The model under review builds one solid part; all positions refer to its coordinate system, in mm. A direction names the side the tool comes from. Give positions to 0.01 mm unless a question says otherwise; leave off trailing zeros. Loops run counter-clockwise (first coordinate to the right, second up) from the corner with the lowest first, then second, coordinate; pieces in that order, holes last. Notation, with made-up numbers: (72.5, 37) - (108.5, 37) arc R28 ccw to (108.5, 68) - close; hole circle Ø2 at (40.25, 51). An arc over 180 degrees is marked (long way). Answer as a JSON object with one key per item and string values.
from build123d import *

# Parameters (mm, degrees)
SKETCH4_W            = 31.4
SKETCH4_H            = 31.4
SKETCH4_W_2          = 25.4
SKETCH4_H_2          = 25.4
BOSS_EXTRUDE3_DEPTH  = 30
SKETCH5_W            = 31.4
SKETCH5_H            = 31.4
BOSS_EXTRUDE4_DEPTH  = 5
SKETCH6_W            = 31.4
SKETCH6_H            = 8
BOSS_EXTRUDE5_DEPTH  = 5
BOSS_EXTRUDE6_DEPTH  = 8
SKETCH8_R            = 9.5
BOSS_EXTRUDE7_DEPTH  = 8
SKETCH9_W            = 31.4
SKETCH9_H            = 10
BOSS_EXTRUDE8_DEPTH  = 5
SKETCH10_W           = 31.4
SKETCH10_H           = 10
BOSS_EXTRUDE9_DEPTH  = 11
SKETCH11_W           = 5.2
SKETCH11_H           = 10
BOSS_EXTRUDE10_DEPTH = 40
BOSS_EXTRUDE11_DEPTH = 3
CUT_EXTRUDE1_START   = 8
SKETCH8_2_R          = 9.5
CUT_EXTRUDE1_DEPTH   = 24
SKETCH14_W           = 21
SKETCH14_H           = 13
CUT_EXTRUDE2_DEPTH   = 2


with BuildPart() as part:
    # Sketch4 → Boss-Extrude3 (new body)
    with BuildSketch(Plane.XY):
        Rectangle(SKETCH4_W, SKETCH4_H)
        Rectangle(SKETCH4_W_2, SKETCH4_H_2, mode=Mode.SUBTRACT)
    extrude(amount=BOSS_EXTRUDE3_DEPTH)

    # Sketch5 → Boss-Extrude4 (add)
    with BuildSketch(Plane.XY.offset(30)):
        Rectangle(SKETCH5_W, SKETCH5_H)
    extrude(amount=BOSS_EXTRUDE4_DEPTH)

    # Sketch6 → Boss-Extrude5 (add)
    with BuildSketch(Plane.XY.offset(35)):
        Rectangle(SKETCH6_W, SKETCH6_H)
    extrude(amount=BOSS_EXTRUDE5_DEPTH)

    # Sketch7 → Boss-Extrude6 (add)
    with BuildSketch(Plane.XZ.offset(4)):
        with BuildLine():
            Line((-15.7, 40), (-15.7, 52))
            ThreePointArc((-15.7, 52), (-11.306601718, 62.606601718), (-0.7, 67))
            Line((-0.7, 67), (0.7, 67))
            ThreePointArc((0.7, 67), (11.306601718, 62.606601718), (15.7, 52))
            Line((15.7, 52), (15.7, 40))
            Line((15.7, 40), (-15.7, 40))
        make_face()
    extrude(amount=-BOSS_EXTRUDE6_DEPTH)

    # Sketch8 → Boss-Extrude7 (add)
    with BuildSketch(Plane.XZ.offset(4)):
        with Locations(Location((0, 52, 0), (0, 0, 180))):
            Circle(SKETCH8_R)
    boss_extrude7 = extrude(amount=BOSS_EXTRUDE7_DEPTH)

    # Mirror1: Boss-Extrude7 across plane
    add(boss_extrude7.mirror(Plane.ZX))

    # Sketch9 → Boss-Extrude8 (add)
    with BuildSketch(Plane(origin=(0, 15.7, 0), x_dir=(1, 0, 0), z_dir=(0, 1, 0))):
        with Locations((0, -27)):
            Rectangle(SKETCH9_W, SKETCH9_H)
    extrude(amount=BOSS_EXTRUDE8_DEPTH)

    # Sketch10 → Boss-Extrude9 (add)
    with BuildSketch(Plane(origin=(0, 15.7, 0), x_dir=(1, 0, 0), z_dir=(0, 1, 0))):
        with Locations((0, -17)):
            Rectangle(SKETCH10_W, SKETCH10_H)
    extrude(amount=BOSS_EXTRUDE9_DEPTH)

    # Sketch11 → Boss-Extrude10 (add)
    with BuildSketch(Plane(origin=(0, 20.7, 0), x_dir=(1, 0, 0), z_dir=(0, 1, 0))):
        with Locations((-13.1, -27)):
            Rectangle(SKETCH11_W, SKETCH11_H)
        with Locations((13.1, -27)):
            Rectangle(SKETCH11_W, SKETCH11_H)
    extrude(amount=BOSS_EXTRUDE10_DEPTH)

    # Sketch12 → Boss-Extrude11 (add)
    with BuildSketch(Plane.XY.offset(32)):
        Polygon((-15.7, 60.7), (-10.5, 60.7), (-10.5, 20.7), (10.5, 20.7), (10.5, 60.7), (15.7, 60.7), (15.7, 15.7), (-15.7, 15.7), align=None)
    extrude(amount=BOSS_EXTRUDE11_DEPTH)

    # Sketch8_2 → Cut-Extrude1 (cut)
    with BuildSketch(Plane.XZ.offset(4).offset(CUT_EXTRUDE1_START)):
        with Locations(Location((0, 52, 0), (0, 0, 270))):
            Circle(SKETCH8_2_R)
    extrude(amount=-CUT_EXTRUDE1_DEPTH, mode=Mode.SUBTRACT)

    # Sketch14 → Cut-Extrude2 (cut)
    with BuildSketch(Plane(origin=(0, 20.7, 0), x_dir=(1, 0, 0), z_dir=(0, 1, 0))):
        with Locations((0, -28.5)):
            Rectangle(SKETCH14_W, SKETCH14_H)
    extrude(amount=-CUT_EXTRUDE2_DEPTH, mode=Mode.SUBTRACT)


solid = part.part
Q1. To check wall thickness, follow probe 1 along Y at (x, z) = (-3, 29.5); probe 2 along X at (y, z) = (-2, 16.5); probe 3 along Y at (x, z) = (-10, 20). State the ranges of each line that lie inside material, in increasing order. Write a range as [from, to].
Results:
{"probe 1": "y = [-15.7, -12.7], [12.7, 18.7]", "probe 2": "x = [-15.7, -12.7], [12.7, 15.7]", "probe 3": "y = [-15.7, -12.7], [12.7, 26.7]"}
Q2. Consider section D-D, the plane y = 47.5. State the section outline as (x, z) points, plus the area to 3 significant figures.
Results:
{"outline": "(-15.7, 22) - (-10.5, 22) - (-10.5, 35) - (-15.7, 35) - close; (10.5, 22) - (15.7, 22) - (15.7, 35) - (10.5, 35) - close", "area": "135 mm^2"}
Q3. For faces 1 (the face through (13, 43, 22)), 2 (the face through (0, 23, 22)), 3 (the face through (0, -10, 35)), 4 (the face through (0, -12.7, 15)), list the 3-axis set-ups (+Z, -Z, +X, -X, +Y, -Y) from which the entire face can be reached by the end or side of a thin tool; tool diameter is ignored.
Results:
{"face 1": "-Z, +X, -X, +Y", "face 2": "+Z, +Y", "face 3": "+Z, +X, -X, -Y", "face 4": "-Z"}
Q4. Consider section A-A, the plane z = 13.5. State the section outline as (x, y) points, plus the area to 3 significant figures.
Results:
{"outline": "(-15.7, -15.7) - (15.7, -15.7) - (15.7, 26.7) - (-15.7, 26.7) - close; hole (-12.7, -12.7) - (12.7, -12.7) - (12.7, 12.7) - (-12.7, 12.7) - close", "area": "686 mm^2"}
Q5. Clearance check with flat-ended pins moving along their axes: pin 1 Ø7.5 at (x, y) = (5.5, 0.5) entering from -Z; pin 2 Ø12 at (x, y) = (-1.5, 21) entering from -Z; pin 3 Ø6 at (x, y) = (-2.5, -11) entering from +Z; pin 4 Ø6.5 at (x, y) = (-1.5, 22) entering from +Z. State where each tip first meets the part, or that it passes through.
Results:
{"pin 1": "stops at z = 30", "pin 2": "stops at z = 0", "pin 3": "stops at z = 35", "pin 4": "stops at z = 22"}
Q6. Consider section B-B, the plane y = 2.5. State the section outline as (x, z) points, plus the area to 3 significant figures.
Results:
{"outline": "(-15.7, 0) - (-12.7, 0) - (-12.7, 30) - (12.7, 30) - (12.7, 0) - (15.7, 0) - (15.7, 52) arc R15 ccw to (0.7, 67) - (-0.7, 67) arc R15 ccw to (-15.7, 52) - close; hole circle Ø19 at (0, 52)", "area": "962 mm^2"}
Q7. Consider section C-C, the plane x = -2.5. State the section outline as (y, z) points, plus the area to 3 significant figures.
Results:
{"outline": "(-15.7, 0) - (-12.7, 0) - (-12.7, 30) - (12.7, 30) - (12.7, 0) - (15.7, 0) - (15.7, 12) - (26.7, 12) - (26.7, 22) - (18.7, 22) - (18.7, 35) - (4, 35) - (4, 42.83) - (-4, 42.83) - (-4, 35) - (-15.7, 35) - close; (-4, 61.17) - (4, 61.17) - (4, 66.89) - (-4, 66.89) - close", "area": "594 mm^2"}
Q8. The part is to be moulded in two halves that separate along X. For faces 5 (the face through (0, 15.7, 6)), 6 (the face through (-10.5, 40, 28)), 7 (the face through (-11.42, -0.06, 62.49)), 8 (the face through (-12.7, 0, 15)), say which applies: +X half, -X half, draft (parallel to the pull), parting line (faces both ways), or undercut.
Results:
{"face 5": "draft", "face 6": "undercut", "face 7": "-X half", "face 8": "undercut"}
